Check sheet for the modelled part. Datum: model origin and axes. Units: mm. A direction names the side the tool comes from. Coordinates: 2 decimals unless noted, no trailing zeros. Write each loop counter-clockwise with the first axis right and the second up, starting at its lowest first coordinate (ties: lowest second). Pieces come first, ordered by that corner, then holes. Notation, with made-up numbers: (86, 74) - (112, 74) arc R13 cw to (112, 79) - close; hole circle Ø5 at (23.25, -34). An arc over 180 degrees is marked (long way). Answer as CSV lines item,"result". Start each with the question number.
from build123d import *

# Parameters (mm, degrees)
F0_W     = 39.643229451
F0_H     = 62.91637104
F1_DEPTH = 3
F2_R     = 5
F3_R     = 1.2078964804
F3_R_2   = 1.1945278086
F3_R_3   = 1.7688403941
F3_R_4   = 5.8693557263
F3_R_5   = 3.6035226858
F3_R_6   = 3.4212098418
F5_DEPTH = 3
F6_DEPTH = 5


# Not quite as in the source:
# - the program builds the solid bodies; features that only make, move or delete a surface that nothing else refers to are left out


with BuildPart() as f1:
    # F0 (on Front) → F1 (new body)
    with BuildSketch(Plane.XZ):
        with Locations((-25.5412899423, 17.5534696318)):
            Rectangle(F0_W, F0_H)
    extrude(amount=F1_DEPTH)

    # F2
    f2_edges = [f1.edges().sort_by_distance(p)[0] for p in [
        (-45.362905, -1.5, 49.011655),
        (-45.362905, -1.5, -13.904716),
        (-5.719675, -1.5, -13.904716),
        (-5.719675, -1.5, 49.011655),
    ]]
    fillet(f2_edges, radius=F2_R)

    # F3 (on face) → F5 (join)
    with BuildSketch(Plane(origin=(0, 0, 0), x_dir=(-1, 0, 0), z_dir=(0, 1, 0))):
        with Locations((38.1972528994, 45.2637411654)):
            Circle(F3_R)
        with Locations((35.0141488016, 44.0116551518)):
            Circle(F3_R_2)
        with Locations((30.9397745878, 45.2637411654)):
            Circle(F3_R_3)
        with Locations((23.9369440824, 35.4597829282)):
            Circle(F3_R_4)
        with Locations((35.1414717734, 35.7144325972)):
            Circle(F3_R_5)
        with Locations((10.6952302158, 35.7144325972)):
            Circle(F3_R_6)
    extrude(amount=F5_DEPTH)

    # F6 (add): a face of the model
    f6_faces = [f1.faces().sort_by_distance(p)[0] for p in [
        (-25.6181685943, 0, 15.8495495724),
    ]]
    extrude(f6_faces, amount=F6_DEPTH)


solid = f1.part
(1) Go/stop test with flat-tipped pins: P1, Ø8.5, axis at x = -35.14, z = 35.71, coming from the +Y side; P2, Ø2, axis at x = -10.5, z = 34.5, coming from the +Y side. Record where each tip stops, or that it passes through.
(2) Release check for a two-part mould opening along X. For faces 1 (the face through (-31.54, 3.99, 35.87)), 2 (the face through (-7.15, 0.94, 47.51)), 3 (the face through (-45.363, 1, 17)), 4 (the face through (-26, 5, 18)) record: pulls with the +X half, pulls with the -X half, needs draft (parallel to the pull), parting line crosses it, or undercut.
(3) Cross-section at C-C on x = -19.5. Record the boundary of the cut face in (y, z), plus the area to 3 significant figures.
(4) Tool access check on faces 5 (the face through (-35, 3, 36)), 6 (the face through (-7.223, 0.944, -12.479)). Record the directions out of +Z, -Z, +X, -X, +Y, -Y that give a thin tool (end or side, any length) a straight path to the whole face; none if there is none.
(5) Cross-section at D-D on x = -38. Record the boundary of the cut face in (y, z), plus the area to 3 significant figures.
(6) Material ranges on probe 1 along Z at (x, y) = (-37.5, 4.25); probe 2 along Y at (x, z) = (-27.5, 33.5); probe 3 along X at (y, z) = (4, 31.5), recorded low to high. Write a range as from..to.
(7) Cross-section at A-A on y = 4. Record the boundary of the cut face in (x, z) (3 decimals), plus the area to 3 significant figures.
(8) Cross-section at B-B on x = -26. Record the boundary of the cut face in (y, z).
Checked values:
1,P1,"y = 5"
1,P2,"y = 3"
2,face 1,"undercut"
2,face 2,"pulls with the +X half"
2,face 3,"pulls with the -X half"
2,face 4,"needs draft"
3,outline,"(-3, -13.9) - (5, -13.9) - (5, 31.62) - (3, 31.62) - (3, 39.3) - (5, 39.3) - (5, 49.01) - (-3, 49.01) - close"
3,area,"488 mm^2"
4,face 5,"+Y"
4,face 6,"-Z, +X, +Y, -Y"
5,outline,"(-3, -13.9) - (5, -13.9) - (5, 33.52) - (3, 33.52) - (3, 37.91) - (5, 37.91) - (5, 44.07) - (3, 44.07) - (3, 46.46) - (5, 46.46) - (5, 49.01) - (-3, 49.01) - close"
5,area,"490 mm^2"
6,probe 1,"-13.9..32.99, 38.44..44.28, 46.25..49.01"
6,probe 2,"-3..3"
6,probe 3,"-45.36..-28.27, -19.6..-5.72"
7,outline,"(-45.363, -8.905) arc R5 ccw to (-40.363, -13.905) - (-10.72, -13.905) arc R5 ccw to (-5.72, -8.905) - (-5.72, 44.012) arc R5 ccw to (-10.72, 49.012) - (-40.363, 49.012) arc R5 ccw to (-45.363, 44.012) - close; hole circle Ø2.416 at (-38.197, 45.264); hole circle Ø7.207 at (-35.141, 35.714); hole circle Ø2.389 at (-35.014, 44.012); hole circle Ø3.538 at (-30.94, 45.264); hole circle Ø11.739 at (-23.937, 35.46); hole circle Ø6.842 at (-10.695, 35.714)"
7,area,"2,270 mm^2"
8,outline,"(-3, -13.9) - (5, -13.9) - (5, 29.96) - (3, 29.96) - (3, 40.95) - (5, 40.95) - (5, 49.01) - (-3, 49.01) - close"
